Geometry check sheet. Reference: the model listing, model coordinates, mm. Face numbers are marked on the shaded views. A direction names the side the tool comes from. Give positions to 0.01 mm unless a question says otherwise; leave off trailing zeros. Order: outer loops, then holes, each group sorted by start corner. A loop starts at its lowest first (then second) coordinate and runs counter-clockwise, first axis right, second up. Notation, with made-up numbers: M 87.5,10 L 139.5,10 A12 ccw 139.5,30 Z; hole C 12.25,-39.75 d1. An arc over 180 degrees is marked long. Use CSV: the item, a comma, the result in double quotes. Start each with the question number.
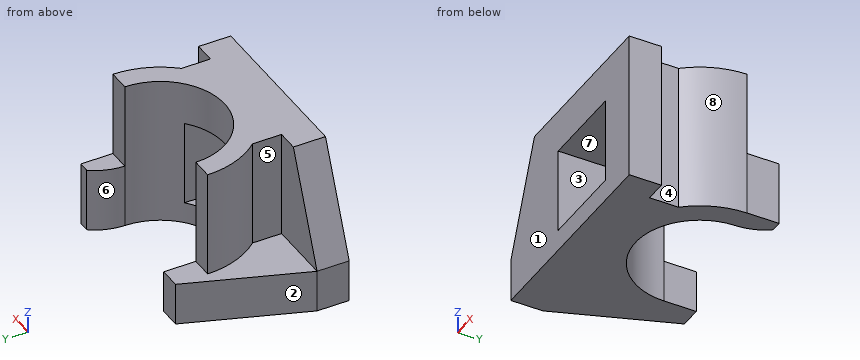
from build123d import *

# Parameters (mm, degrees)
BOSS_EXTRUDE1_DEPTH = 15
BOSS_EXTRUDE2_DEPTH = 70
BOSS_EXTRUDE3_DEPTH = 20
BOSS_EXTRUDE4_DEPTH = 30
CUT_EXTRUDE1_DEPTH  = 116.758369028
SKETCH6_W           = 40
SKETCH6_H           = 40
CUT_EXTRUDE2_DEPTH  = 116.758369028


with BuildPart() as part:
    # Sketch1 → Boss-Extrude1 (new body)
    with BuildSketch(Plane(origin=(0, 0, 0), x_dir=(1, 0, 0), z_dir=(0, 1, 0))):
        Polygon((-60, 0), (40, 0), (40, -70), (-40, -70), (-60, -20), align=None)
    extrude(amount=BOSS_EXTRUDE1_DEPTH)

    # Sketch2 → Boss-Extrude2 (add)
    with BuildSketch(Plane.XY):
        with BuildLine():
            Line((-30, 10), (30, 10))
            Line((30, 10), (30, 28.542486889))
            ThreePointArc((30, 28.542486889), (37.416573868, 40.857864376), (40, 55))
            Line((40, 55), (-40, 55))
            ThreePointArc((-40, 55), (-37.416573868, 40.857864376), (-30, 28.542486889))
            Line((-30, 28.542486889), (-30, 10))
        make_face()
    extrude(amount=BOSS_EXTRUDE2_DEPTH)

    # Sketch3 → Boss-Extrude3 (add)
    with BuildSketch(Plane.XY):
        Polygon((-60, 15), (-30, 15), (-30, 70), (-40, 70), align=None)
    extrude(amount=BOSS_EXTRUDE3_DEPTH)

    # Sketch4 → Boss-Extrude4 (add)
    with BuildSketch(Plane.XY):
        with BuildLine():
            Line((30, 55), (40, 55))
            Line((40, 55), (40, 70))
            Line((40, 70), (35, 70))
            ThreePointArc((35, 70), (31.282917549, 62.90569415), (30, 55))
        make_face()
    extrude(amount=BOSS_EXTRUDE4_DEPTH)

    # Sketch5 → Cut-Extrude1 (cut, through all)
    with BuildSketch(Plane.XY):
        with BuildLine():
            Line((-30, 55), (30, 55))
            ThreePointArc((30, 55), (0, 25), (-30, 55))
        make_face()
    extrude(amount=CUT_EXTRUDE1_DEPTH, mode=Mode.SUBTRACT)

    # Sketch6 → Cut-Extrude2 (cut, through all)
    with BuildSketch(Plane(origin=(0, 0, 0), x_dir=(1, 0, 0), z_dir=(0, 1, 0))):
        with Locations((0, -30)):
            Rectangle(SKETCH6_W, SKETCH6_H)
    extrude(amount=CUT_EXTRUDE2_DEPTH, mode=Mode.SUBTRACT)


solid = part.part
(1) Draft check along Y on the marked faces 1, 2, 3 and 4. Enter one of: +Y half, -Y half, draft (parallel to the pull), parting line (faces both ways), or undercut.
(2) Go/stop test with flat-tipped pins: P1, Ø5, axis at x = -34, z = 48.5, coming from the +Y side; P2, Ø1, axis at x = -46.5, y = 29, coming from the -Z side; P3, Ø5, axis at y = 44.5, z = 50.5, coming from the +X side; P4, Ø8, axis at y = 32, z = 21, coming from the -X side. Record where each tip stops, or that it passes through.
(3) Sectioned sample at C-C on z = 17.5. Record the cut outline in (x, y), then the cut area to 3 significant figures.
(4) Sectioned sample at D-D on y = 38. Record the cut outline in (x, z).
(5) Sectioned sample at B-B on y = 5. Record the cut outline in (x, z).
(6) Access from +Z, -Z, +X, -X, +Y, -Y to the whole of each face (thin tool, end or side, straight path). Record for the marked faces 5, 6, 7 and 8.
(7) Sectioned sample at A-A on x = 0. Record the cut outline in (y, z).
(8) Thickness scan on line 1 (Z direction, x = -2, y = 10); line 2 (X direction, y = 12.5, z = 17); line 3 (X direction, y = 22, z = 35). Record the ranges inside material, lowest first.
Responses:
1,face 1,"-Y half"
1,face 2,"+Y half"
1,face 3,"draft"
1,face 4,"undercut"
2,P1,"y = 55"
2,P2,"z = 0"
2,P3,"x = 39.19"
2,P4,"x = -55.23"
3,outline,"M -60,0 L -20,0 L -20,32.64 A30 cw -30,55 L -30,70 L -40,70 L -60,15 Z; M 20,0 L 40,0 L 40,15 L 30,15 L 30,28.54 A40 ccw 40,55 L 40,70 L 35,70 A25 ccw 30,55 A30 cw 20,32.64 Z"
3,area,"2,800 mm2"
4,outline,"M -51.64,0 L -24.72,0 L -24.72,70 L -36.21,70 L -36.21,20 L -51.64,20 Z; M 24.72,0 L 36.21,0 L 36.21,70 L 24.72,70 Z"
5,outline,"M -60,0 L 40,0 L 40,70 L -40,70 L -60,20 Z; hole M -20,10 L 20,10 L 20,50 L -20,50 Z"
6,face 5,"+Z, -X"
6,face 6,"+Z, -Z, +Y"
6,face 7,"+Y, -Y"
6,face 8,"+Z, -Z, +X"
7,outline,"M 0,0 L 25,0 L 25,10 L 0,10 Z; M 0,50 L 25,50 L 25,70 L 0,70 Z"
8,line 1,"0 to 10, 50 to 70"
8,line 2,"-60 to -20, 20 to 40"
8,line 3,"-30 to -20, 20 to 30"
